from build123d import *

# Parameters (mm, degrees)
SKETCH_1_W          = 85
SKETCH_1_H          = 102
EXTRUDE_1_DEPTH     = 6
CUT_EXTRUDE_1_DEPTH = 75.861411438
SKETCH_3_R          = 4
CUT_EXTRUDE_2_DEPTH = 75.861411438
SKETCH_4_W          = 20
SKETCH_4_H          = 18
CUT_EXTRUDE_3_DEPTH = 75.861411438


with BuildPart() as part:
    # Эскиз1 → Вытянуть1 (new body)
    with BuildSketch(Plane(origin=(0, 0, 0), x_dir=(1, 0, 0), z_dir=(0, 1, 0))):
        with Locations((0, -10.334989382)):
            Rectangle(SKETCH_1_W, SKETCH_1_H)
    extrude(amount=EXTRUDE_1_DEPTH)

    # Эскиз2 → Вырез-Вытянуть1 (cut, through all)
    with BuildSketch(Plane(origin=(0, 6, 0), x_dir=(1, 0, 0), z_dir=(0, 1, 0))):
        Polygon((42.5, 3.665010618), (20, 40.665010618), (42.5, 40.665010618), align=None)
        Polygon((-42.5, 40.665010618), (-42.5, 3.665010618), (-20, 40.665010618), align=None)
    extrude(amount=-CUT_EXTRUDE_1_DEPTH, mode=Mode.SUBTRACT)

    # Эскиз3 → Вырез-Вытянуть2 (cut, through all)
    with BuildSketch(Plane(origin=(0, 6, 0), x_dir=(1, 0, 0), z_dir=(0, 1, 0))):
        with Locations(Location((0, -28.834989382, 0), (0, 0, 270))):
            Circle(SKETCH_3_R)
    extrude(amount=-CUT_EXTRUDE_2_DEPTH, mode=Mode.SUBTRACT)

    # Эскиз4 → Вырез-Вытянуть3 (cut, through all)
    with BuildSketch(Plane(origin=(0, 6, 0), x_dir=(1, 0, 0), z_dir=(0, 1, 0))):
        with Locations((3.2e-08, 31.665010618)):
            Rectangle(SKETCH_4_W, SKETCH_4_H)
    extrude(amount=-CUT_EXTRUDE_3_DEPTH, mode=Mode.SUBTRACT)


solid = part.part
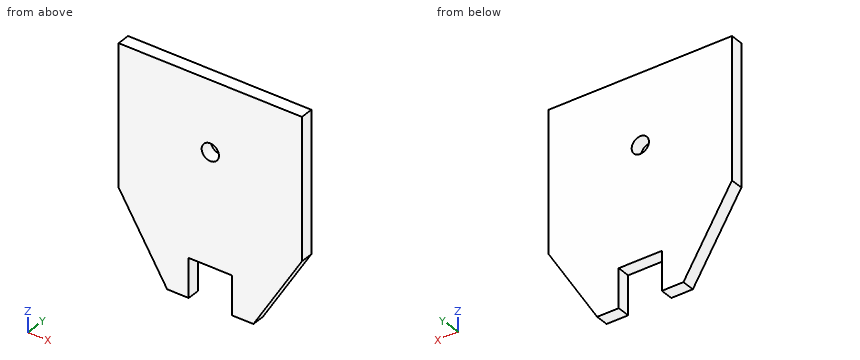
Model file for the job. Use its own axes, mm. Coordinates: 2 decimals unless noted, no trailing zeros. Loops run counter-clockwise (first coordinate to the right, second up) from the corner with the lowest first, then second, coordinate; pieces in that order, holes last. Notation, with made-up numbers: (27.25, 63.5) -> (58.25, 63.5) arc R34 ccw to (58.25, 99.5) -> close; hole circle Ø11 at (66, 62). An arc over 180 degrees is marked (long way). Use one line per item in the form item = value. Start each with the question number.
(1) Cut at A-A on x = 0. Give the cut face in (y, z).
(2) Cut at D-D on z = -19.5. Give the cut face in (x, y).
(3) Probe probe 1 along Z at (x, y) = (38, 2.95); probe 2 along Z at (x, y) = (0.5, 4.2); probe 3 along Z at (x, y) = (32, 4.4). List the from-to ranges inside material, lowest first. Write a range as from..to.
(4) Cut at B-B on y = 2.9. Give the cut face in (x, z).
(5) Cut at C-C on z = 30. Give the cut face in (x, y), and give its area (3 significant figures).
(6) Flat gauge pins, fed straight in: pin 1 (6 mm diameter, centred on x = 28, z = -8, fed in from -Y); pin 2 (1.8 mm diameter, centred on y = 2, z = -30.5, fed in from +X). Where does each tip first touch, or does it go through?
Values:
q1.outline = (0, -22.67) -> (6, -22.67) -> (6, 24.83) -> (0, 24.83) -> close; (0, 32.83) -> (6, 32.83) -> (6, 61.33) -> (0, 61.33) -> close
q2.outline = (-32.87, 0) -> (32.87, 0) -> (32.87, 6) -> (-32.87, 6) -> close
q3.probe_1 = -11.07..61.33
q3.probe_2 = -22.67..24.87, 32.8..61.33
q3.probe_3 = -20.93..61.33
q4.outline = (-42.5, -3.67) -> (-20, -40.67) -> (-10, -40.67) -> (-10, -22.67) -> (10, -22.67) -> (10, -40.67) -> (20, -40.67) -> (42.5, -3.67) -> (42.5, 61.33) -> (-42.5, 61.33) -> close; hole circle Ø8 at (0, 28.83)
q5.outline = (-42.5, 0) -> (-3.83, 0) -> (-3.83, 6) -> (-42.5, 6) -> close; (3.83, 0) -> (42.5, 0) -> (42.5, 6) -> (3.83, 6) -> close
q5.area = 464 mm2
q6.pin_1 = 0
q6.pin_2 = 26.73
